from build123d import *

# Parameters (mm, degrees)
SKETCH_1_W               = 20
SKETCH_1_H               = 20
EXTRUDE_1_DEPTH          = 17
SKETCH_2_W               = 16.8
SKETCH_2_H               = 12.6
CUT_EXTRUDE_1_DEPTH      = 16.8
CUT_EXTRUDE_2_DEPTH      = 16.8
CUT_EXTRUDE_2_DEPTH_BACK = 16.8
CUT_EXTRUDE_3_DEPTH      = 16.8


with BuildPart() as part:
    # 草图1 → 凸台-拉伸1 (new body)
    with BuildSketch(Plane.XY):
        Rectangle(SKETCH_1_W, SKETCH_1_H)
    extrude(amount=EXTRUDE_1_DEPTH)

    # 草图2 → 切除-拉伸1 (cut)
    with BuildSketch(Plane(origin=(0, 10, 0), x_dir=(1, 0, 0), z_dir=(0, 1, 0))):
        with Locations((1.6, -8.5)):
            Rectangle(SKETCH_2_W, SKETCH_2_H)
    extrude(amount=-CUT_EXTRUDE_1_DEPTH, mode=Mode.SUBTRACT)

    # 草图3 → 切除-拉伸2 (cut, two sides: drawn at the far end of the back side and taken through both)
    with BuildSketch(Plane.XY.offset(2.2).offset(-CUT_EXTRUDE_2_DEPTH_BACK)):
        Polygon((-6.8, 10), (10, -6.8), (10, 10), align=None)
    extrude(amount=CUT_EXTRUDE_2_DEPTH + CUT_EXTRUDE_2_DEPTH_BACK, mode=Mode.SUBTRACT)

    # 草图4 → 切除-拉伸3 (cut)
    with BuildSketch(Plane(origin=(-6.8, 0, 0), x_dir=(0, 0, -1), z_dir=(1, 0, 0))):
        with BuildLine():
            Line((-5.4, 0.2), (-5.4, 3))
            ThreePointArc((-5.4, 3), (-8.5, 6.1), (-11.6, 3))
            Line((-11.6, 3), (-11.6, 0.2))
            ThreePointArc((-11.6, 0.2), (-8.5, -2.9), (-5.4, 0.2))
        make_face()
    cut_extrude_3 = extrude(amount=-CUT_EXTRUDE_3_DEPTH, mode=Mode.SUBTRACT)

    # 镜向1: 切除-拉伸3 across plane
    add(cut_extrude_3.mirror(Plane(origin=(0, 0, 0), x_dir=(0, 0, 1), z_dir=(0.7071067811865479, -0.7071067811865471, 0))), mode=Mode.SUBTRACT)


solid = part.part
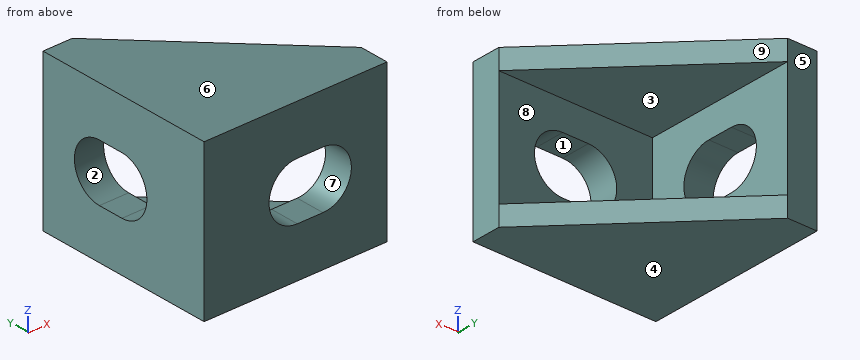
Verification items for the finished model (mm, model axes). Face numbers are marked on the shaded views. A direction names the side the tool comes from. Coordinates: 2 decimals unless noted, no trailing zeros. Write each loop counter-clockwise with the first axis right and the second up, starting at its lowest first coordinate (ties: lowest second). Pieces come first, ordered by that corner, then holes. Notation, with made-up numbers: (13, -37) -> (35, -37) arc R25 ccw to (35, -3) -> close; hole circle Ø9 at (-37.5, -35). An arc over 180 degrees is marked (long way). One line per item, written item: value. Start each with the question number.
Q1. Cross-section at C-C on z = 8.5. Enter the section's corners in (x, y).
Q2. Cross-section at D-D on y = -5.75. Enter the section's corners in (x, z).
Q3. Cross-section at B-B on y = 2. Enter the section's corners in (x, z), and give its area (3 significant figures).
Q4. Mould release check, pull along Z, two halves, no side actions. Record for the marked faces 6, 7, 8 and 9: pulls with the +Z half, pulls with the -Z half, needs draft (parallel to the pull), parting line crosses it, or undercut.
Q5. Go/stop test with flat-tipped pins: P1, Ø2, axis at x = 4.5, z = 2.5, coming from the +Y side; P2, Ø1.5, axis at x = -7, y = 3.5, coming from the -Z side; P3, Ø4, axis at x = -4, z = 15, coming from the +Y side; P4, Ø6.5, axis at x = 5.5, z = 11, coming from the +Y side. Record where each tip stops, or that it passes through.
Q6. Cross-section at A-A on x = 0.75. Enter the section's corners in (y, z).
Q7. Thickness scan on L1, parallel to Z at x = -4.5, y = 2.5; L2, parallel to X at y = 1.25, z = 13; L3, parallel to Z at x = -2.25, y = -8. Record the ranges inside material, lowest first. Write a range as from..to.
Q8. Access from +Z, -Z, +X, -X, +Y, -Y to the whole of each face (thin tool, end or side, straight path). Record for the marked faces 1, 2, 3, 4 and 5.
Checked values:
1. outline: (-10, -10) -> (-2.9, -10) -> (-2.9, -6.8) -> (-6.8, -6.8) -> (-6.8, -2.9) -> (-10, -2.9) -> close; (-10, 6.1) -> (-6.8, 6.1) -> (-6.8, 10) -> (-10, 10) -> close; (6.1, -10) -> (10, -10) -> (10, -6.8) -> (6.1, -6.8) -> close
2. outline: (-10, 0) -> (8.95, 0) -> (8.95, 2.2) -> (-6.8, 2.2) -> (-6.8, 14.8) -> (8.95, 14.8) -> (8.95, 17) -> (-10, 17) -> close
3. outline: (-10, 0) -> (1.2, 0) -> (1.2, 2.2) -> (-6.8, 2.2) -> (-6.8, 5.4) -> (-10, 5.4) -> close; (-10, 11.6) -> (-6.8, 11.6) -> (-6.8, 14.8) -> (1.2, 14.8) -> (1.2, 17) -> (-10, 17) -> close
3. area: 69.8 mm²
4. face 6: pulls with the +Z half
4. face 7: undercut
4. face 8: undercut
4. face 9: needs draft
5. P1: stops at y = -0.35
5. P2: stops at z = 0
5. P3: stops at y = 9.2
5. P4: stops at y = -6.8
6. outline: (-10, 0) -> (2.45, 0) -> (2.45, 2.2) -> (-6.8, 2.2) -> (-6.8, 5.4) -> (-10, 5.4) -> close; (-10, 11.6) -> (-6.8, 11.6) -> (-6.8, 14.8) -> (2.45, 14.8) -> (2.45, 17) -> (-10, 17) -> close
7. L1: z = 0..2.2, 14.8..17
7. L2: x = -10..-6.8
7. L3: z = 0..6.6, 10.4..17
8. face 1: +Y, -Y
8. face 2: +X, -X
8. face 3: +X, +Y
8. face 4: -Z, +X, -X, +Y, -Y
8. face 5: +Z, -Z, +X, -X, +Y
